```python
from build123d import *

# Parameters (mm, degrees)
F1_DEPTH = 25.4
F2_W     = 6.35
F2_H     = 12.7
F3_DEPTH = 6.35
F4_W     = 19.05
F4_H     = 12.7
F5_DEPTH = 12.701


with BuildPart() as f1:
    # F0 (on Front) → F1 (new body)
    with BuildSketch(Plane.XZ):
        Polygon((0, 25.4), (0, 0), (33.02, 0), (33.02, 12.7), (6.35, 12.7), (6.35, 25.4), align=None)
    extrude(amount=F1_DEPTH)

    # F2 (on face) → F3 (cut)
    with BuildSketch(Plane.XZ.offset(25.4)):
        with Locations((3.175, 19.05)):
            Rectangle(F2_W, F2_H)
    extrude(amount=-F3_DEPTH, mode=Mode.SUBTRACT)

    # F4 (on face) → F5 (cut, through all)
    with BuildSketch(Plane.XY.offset(12.7)):
        with Locations((23.495, -19.05)):
            Rectangle(F4_W, F4_H)
    extrude(amount=-F5_DEPTH, mode=Mode.SUBTRACT)


solid = f1.part
```
Geometry: final body of the model. Coordinates: model frame, mm. A direction names the side the tool comes from. Coordinates: 2 decimals unless noted, no trailing zeros. Loops run counter-clockwise (first coordinate to the right, second up) from the corner with the lowest first, then second, coordinate; pieces in that order, holes last. Notation, with made-up numbers: M 62,72 L 106,72 A27 ccw 106,88 Z; hole C -13.75,28 d10. An arc over 180 degrees is marked long. Put each result on its own line as item: value.
(1) Cut plane D-D on y = -20. Return the cut outline in (x, z), then the cut area to 3 significant figures.
Answer sheet:
outline: M 0,0 L 13.97,0 L 13.97,12.7 L 0,12.7 Z
area: 177 mm^2
(2) Cut plane B-B on y = -13.75. Return the cut outline in (x, z), then the cut area to 3 significant figures.
Answer sheet:
outline: M 0,0 L 13.97,0 L 13.97,12.7 L 6.35,12.7 L 6.35,25.4 L 0,25.4 Z
area: 258 mm^2
(3) Material intervals for probe 1 along Z at (x, y) = (28.5, -5.75); probe 2 along X at (y, z) = (-17.75, 24.75); probe 3 along Y at (x, z) = (28.5, 1.25), sorted ascending.
Answer sheet:
probe 1: z = 0 to 12.7
probe 2: x = 0 to 6.35
probe 3: y = -12.7 to 0
(4) Access query for faces 1 (the face through (23, -12.7, 6)), 2 (the face through (13, -10, 0)), 3 (the face through (7, -25.4, 6)), 4 (the face through (6.35, -9, 19)), 5 (the face through (3, -19.05, 19)). Directions: +Z, -Z, +X, -X, +Y, -Y. A direction counts if a zero-diameter tool reaches every point of the face in a straight line with its end or side. Return the directions, or none.
Answer sheet:
face 1: +Z, -Z, +X, -Y
face 2: -Z, +X, -X, +Y, -Y
face 3: +Z, -Z, +X, -X, -Y
face 4: +Z, +X, +Y, -Y
face 5: +Z, +X, -X, -Y
(5) Cut plane A-A on z = 7.5. Return the cut outline in (x, y).
Answer sheet:
outline: M 0,-25.4 L 13.97,-25.4 L 13.97,-12.7 L 33.02,-12.7 L 33.02,0 L 0,0 Z
(6) Cut plane C-C on x = 11.5. Return the cut outline in (y, z), then the cut area to 3 significant figures.
Answer sheet:
outline: M -25.4,0 L 0,0 L 0,12.7 L -25.4,12.7 Z
area: 323 mm^2
(7) First-contact query: pin 1 (4 mm diameter, centred on y = -14, z = 17.5, fed in from +X); pin 2 (7 mm diameter, centred on x = 3.5, z = 20.5, fed in from -Y); pin 3 (4 mm diameter, centred on x = 20, z = 6.5, fed in from -Y). Flat tips, straight axial feed; report the tip coordinate or a pass-through.
Answer sheet:
pin 1: stops at x = 6.35
pin 2: stops at y = -19.05
pin 3: stops at y = -12.7
